```python
from build123d import *

# Parameters (mm, degrees)
F0_R     = 9.45
F0_R_2   = 8.65
F1_DEPTH = 8
F2_R     = 8.65
F3_DEPTH = 0.8


# Not quite as in the source:
# - a fillet or chamfer that OpenCascade refuses, or shapes differently, is made with other operations: its cross-section is extruded or revolved along the edge and cut away or added


with BuildPart() as f1:
    # F0 (on Front) → F1 (new body)
    with BuildSketch(Plane.XZ):
        Circle(F0_R)
        Circle(F0_R_2, mode=Mode.SUBTRACT)
    extrude(amount=F1_DEPTH)

    # F2 (on Front) → F3 (join)
    with BuildSketch(Plane.XZ):
        Circle(F2_R)
    extrude(amount=F3_DEPTH)

    # F4: chamfer of 1 on 1 edges, made by hand

    # F4_s1 → F4_t2 (revolve, cut)
    with BuildSketch(Plane.XY):
        Polygon((9.65, -8), (8.65, -7), (8.65, -8), align=None)
    revolve(axis=Axis((0, -8, 0), (0, -1, 0)), mode=Mode.SUBTRACT)


solid = f1.part
```
Here's how the part is built. I have some questions about the finished solid (model axes, mm). Coordinates: 2 decimals unless noted, no trailing zeros. Loops run counter-clockwise (first coordinate to the right, second up) from the corner with the lowest first, then second, coordinate; pieces in that order, holes last. Notation, with made-up numbers: (36.25, -36.5) -> (67.25, -36.5) arc R12 ccw to (67.25, -28.5) -> close; hole circle Ø2 at (66.25, 72). An arc over 180 degrees is marked (long way). Return JSON: item names as keys, results as strings.
1) I need wall thicknesses on line 1 (Z direction, x = 0, y = -2.5); line 2 (Y direction, x = -6.25, z = 2.25); line 3 (X direction, y = -4, z = -0.75). Which ranges of each line are inside material? Lowest first, please. Write a range as from..to.
Results below:
{"line 1": "-9.45..-8.65, 8.65..9.45", "line 2": "-0.8..0", "line 3": "-9.42..-8.62, 8.62..9.42"}
2) If we section it at B-B, the plane x = 0: Write out the boundary of the cut face in (y, z).
Results below:
{"outline": "(-7.8, -9.45) -> (0, -9.45) -> (0, 9.45) -> (-7.8, 9.45) -> (-7, 8.65) -> (-0.8, 8.65) -> (-0.8, -8.65) -> (-7, -8.65) -> close"}
3) If we section it at C-C, the plane y = -3.5: Write out the boundary of the cut face in (x, z).
Results below:
{"outline": "circle Ø18.9 at (0, 0); hole circle Ø17.3 at (0, 0)"}
4) Thinking about a two-plate mould opening in X: for faces 1 (the face through (0, 0, 0)), 2 (the face through (9.014, -3.845, 2.839)), 3 (the face through (8.25, -3.86, 2.6)), 4 (the face through (0, -0.8, 0)), which applies, +X half, -X half, draft (parallel to the pull), parting line (faces both ways), or undercut?
Results below:
{"face 1": "draft", "face 2": "parting line", "face 3": "undercut", "face 4": "undercut"}
5) If we section it at A-A, the plane z = 0: Write out the boundary of the cut face in (x, y), then the cut area to 3 significant figures.
Results below:
{"outline": "(-9.45, -7.8) -> (-8.65, -7) -> (-8.65, -0.8) -> (8.65, -0.8) -> (8.65, -7) -> (9.45, -7.8) -> (9.45, 0) -> (-9.45, 0) -> close", "area": "25.7 mm²"}
6) Will these pins go through, and if not, where does the flat tip stop? pin 1 (1 mm diameter, centred on y = -1.5, z = 1, fed in from +X); pin 2 (2 mm diameter, centred on x = 5.5, z = -1.5, fed in from +Y); pin 3 (1.5 mm diameter, centred on x = 1, z = -6.5, fed in from -Y); pin 4 (1.5 mm diameter, centred on x = -1.5, y = -3.5, fed in from +Z).
Results below:
{"pin 1": "x = 9.44", "pin 2": "y = 0", "pin 3": "y = -0.8", "pin 4": "z = 9.42"}
